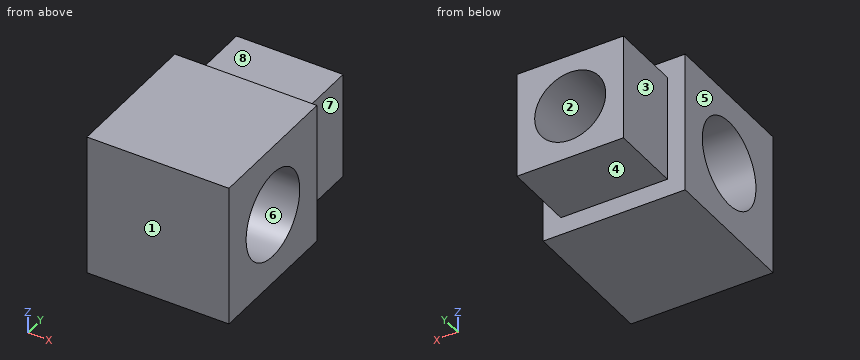
from build123d import *

# Parameters (mm, degrees)
SKETCH1_W           = 20
SKETCH1_H           = 20
SKETCH1_R           = 6.1
BOSS_EXTRUDE1_DEPTH = 10
SKETCH2_W           = 15
SKETCH2_H           = 15
BOSS_EXTRUDE2_DEPTH = 10
SKETCH3_R           = 5
CUT_EXTRUDE1_DEPTH  = 10


with BuildPart() as part:
    # Sketch1 → Boss-Extrude1 (new body, symmetric)
    with BuildSketch(Plane(origin=(0, 0, 0), x_dir=(0, 0, -1), z_dir=(1, 0, 0))):
        Rectangle(SKETCH1_W, SKETCH1_H)
        Circle(SKETCH1_R, mode=Mode.SUBTRACT)
    extrude(amount=BOSS_EXTRUDE1_DEPTH, both=True)

    # Sketch2 → Boss-Extrude2 (add)
    with BuildSketch(Plane(origin=(0, 10, 0), x_dir=(1, 0, 0), z_dir=(0, 1, 0))):
        Rectangle(SKETCH2_W, SKETCH2_H)
    extrude(amount=BOSS_EXTRUDE2_DEPTH)

    # Sketch3 → Cut-Extrude1 (cut)
    with BuildSketch(Plane(origin=(0, 20, 0), x_dir=(1, 0, 0), z_dir=(0, 1, 0))):
        Circle(SKETCH3_R)
    extrude(amount=-CUT_EXTRUDE1_DEPTH, mode=Mode.SUBTRACT)


solid = part.part
The listing builds one solid part. Answer for the finished solid, in the listing's coordinates (mm). Face numbers are marked on the shaded views. A direction names the side the tool comes from. Round coordinates to 2 decimals unless told otherwise and drop trailing zeros. Write each loop counter-clockwise with the first axis right and the second up, starting at its lowest first coordinate (ties: lowest second). Pieces come first, ordered by that corner, then holes. Notation, with made-up numbers: M -18.5,62 L 31.5,62 A20 ccw 31.5,86 Z; hole C 8,-27 d1. An arc over 180 degrees is marked long. Write each question's results on one line, items separated by ' | '. Start each with the question number.
Item 1: Straight lines are drawn through the part: probe 1 along Y at (x, z) = (6.75, -0.25); probe 2 along X at (y, z) = (16.5, 0); probe 3 along Y at (x, z) = (2.5, 0). For each, find the intervals that lie inside material, in ascending order.
Item 2: Given pin 1 Ø8 at (y, z) = (16.5, -2.5) entering from -X; pin 2 Ø8 at (y, z) = (15.5, 2.5) entering from +X; pin 3 Ø3 at (x, y) = (3, 17.5) entering from -Z, each flat-ended and moving along its own axis, determine where each tip first touches the part or whether it passes through.
Item 3: The mould has two halves that part along Z. Classify the marked faces 6, 7 and 8: +Z half, -Z half, draft (parallel to the pull), parting line (faces both ways), or undercut.
Item 4: Find section A-A on y = 0. Write down the section's boundary in (x, z).
Item 5: Which of the six approach directions +Z, -Z, +X, -X, +Y, -Y give full straight-line access (tool end or side, diameter ignored) to the marked faces 1, 2, 3, 4 and 5?
Item 6: Find section D-D on y = 17. Write down the section's boundary in (x, z), and give its area (3 significant figures).
Item 7: Find section C-C on x = 6.75. Write down the section's boundary in (y, z).
Item 8: Find section B-B on z = 0. Write down the section's boundary in (x, y).
Answer block:
1) probe 1: y = -10 to -6.09, 6.09 to 20 | probe 2: x = -7.5 to -5, 5 to 7.5 | probe 3: y = -10 to -6.1, 6.1 to 10
2) pin 1: stops at x = -7.5 | pin 2: stops at x = 7.5 | pin 3: stops at z = -7.5
3) face 6: undercut | face 7: draft | face 8: +Z half
4) outline: M -10,-10 L 10,-10 L 10,-6.1 L -10,-6.1 Z; M -10,6.1 L 10,6.1 L 10,10 L -10,10 Z
5) face 1: +Z, -Z, +X, -X, -Y | face 2: +Y | face 3: +Z, -Z, -X, +Y | face 4: -Z, +X, -X, +Y | face 5: +Z, -Z, -X, +Y, -Y
6) outline: M -7.5,-7.5 L 7.5,-7.5 L 7.5,7.5 L -7.5,7.5 Z; hole C 0,0 d10 | area: 146 mm²
7) outline: M -10,-10 L 10,-10 L 10,-7.5 L 20,-7.5 L 20,7.5 L 10,7.5 L 10,10 L -10,10 Z; hole C 0,0 d12.2
8) outline: M -10,-10 L 10,-10 L 10,-6.1 L -10,-6.1 Z; M -10,6.1 L 10,6.1 L 10,10 L 7.5,10 L 7.5,20 L 5,20 L 5,10 L -5,10 L -5,20 L -7.5,20 L -7.5,10 L -10,10 Z
